from build123d import *

# Parameters (mm, degrees)
SKETCH_2_W          = 130
SKETCH_2_H          = 80
SKETCH_2_R          = 2.5
EXTRUDE_1_DEPTH     = 4.5
SKETCH_4_W          = 80
SKETCH_4_H          = 70
EXTRUDE_2_DEPTH     = 4.5
SKETCH_6_R          = 1.15
CUT_EXTRUDE_2_DEPTH = 4.5
SKETCH_7_R          = 1.15
CUT_EXTRUDE_3_DEPTH = 4.5
SKETCH_8_R          = 1.35
CUT_EXTRUDE_4_DEPTH = 10
SKETCH_9_W          = 40
SKETCH_9_H          = 10
SKETCH_9_W_2        = 30
CUT_EXTRUDE_5_DEPTH = 10
SKETCH_11_W         = 50
SKETCH_11_H         = 30
EXTRUDE_3_DEPTH     = 4.5
SKETCH_12_W         = 20
SKETCH_12_H         = 15
CUT_EXTRUDE_6_DEPTH = 10
SKETCH_13_R         = 2
CUT_EXTRUDE_7_DEPTH = 10
SKETCH_14_R         = 2
CUT_EXTRUDE_8_DEPTH = 10
SKETCH_15_W         = 15
SKETCH_15_H         = 40
CUT_EXTRUDE_9_DEPTH = 10


with BuildPart() as part:
    # 草图2 → 凸台-拉伸1 (new body)
    with BuildSketch(Plane(origin=(0, 0, 0), x_dir=(1, 0, 0), z_dir=(0, 1, 0))):
        with Locations((0, 15)):
            Rectangle(SKETCH_2_W, SKETCH_2_H)
        with Locations(Location((-57, 47, 0), (0, 0, 270))):
            Circle(SKETCH_2_R, mode=Mode.SUBTRACT)
        with Locations(Location((57, 47, 0), (0, 0, 90))):
            Circle(SKETCH_2_R, mode=Mode.SUBTRACT)
        with Locations(Location((57, -17, 0), (0, 0, 270))):
            Circle(SKETCH_2_R, mode=Mode.SUBTRACT)
        with Locations(Location((-57, -17, 0), (0, 0, 90))):
            Circle(SKETCH_2_R, mode=Mode.SUBTRACT)
    extrude(amount=EXTRUDE_1_DEPTH)

    # 草图4 → 凸台-拉伸2 (add)
    with BuildSketch(Plane.XZ):
        with Locations((0, 60)):
            Rectangle(SKETCH_4_W, SKETCH_4_H)
    extrude(amount=-EXTRUDE_2_DEPTH)

    # 草图6 → 切除-拉伸2 (cut)
    with BuildSketch(Plane.XZ):
        with Locations(Location((-31, 5.56384156, 0), (0, 0, 270))):
            Circle(SKETCH_6_R)
        with Locations(Location((31, 5.56384156, 0), (0, 0, 270))):
            Circle(SKETCH_6_R)
    extrude(amount=-CUT_EXTRUDE_2_DEPTH, mode=Mode.SUBTRACT)

    # 草图7 → 切除-拉伸3 (cut)
    with BuildSketch(Plane.XZ):
        with Locations(Location((31, 5.56384156, 0), (0, 0, 270))):
            Circle(SKETCH_7_R)
        with Locations(Location((-25, -51.43615844, 0), (0, 0, 270))):
            Circle(SKETCH_7_R)
        with Locations(Location((25, -51.43615844, 0), (0, 0, 270))):
            Circle(SKETCH_7_R)
    extrude(amount=-CUT_EXTRUDE_3_DEPTH, mode=Mode.SUBTRACT)

    # 草图8 → 切除-拉伸4 (cut)
    with BuildSketch(Plane.XZ):
        with Locations(Location((-21.50477, 84.936614939, 0), (0, 0, 270))):
            Circle(SKETCH_8_R)
        with Locations(Location((36.4733, 84.920764939, 0), (0, 0, 270))):
            Circle(SKETCH_8_R)
        with Locations(Location((36.4823, 35.933764939, 0), (0, 0, 270))):
            Circle(SKETCH_8_R)
        with Locations(Location((-21.5077, 35.922764939, 0), (0, 0, 270))):
            Circle(SKETCH_8_R)
    extrude(amount=-CUT_EXTRUDE_4_DEPTH, mode=Mode.SUBTRACT)

    # 草图9 → 切除-拉伸5 (cut)
    with BuildSketch(Plane.XZ):
        with Locations((0, -5.362073184)):
            Rectangle(SKETCH_9_W, SKETCH_9_H)
        with Locations((0, -28.22464148)):
            Rectangle(SKETCH_9_W, SKETCH_9_H)
        with Locations((7, 71.526054591)):
            Rectangle(SKETCH_9_W_2, SKETCH_9_H)
        with Locations((7, 52.012779739)):
            Rectangle(SKETCH_9_W_2, SKETCH_9_H)
    extrude(amount=-CUT_EXTRUDE_5_DEPTH, mode=Mode.SUBTRACT)

    # 草图11 → 凸台-拉伸3 (add)
    with BuildSketch(Plane.XZ):
        with Locations((0, -70)):
            Rectangle(SKETCH_11_W, SKETCH_11_H)
    extrude(amount=-EXTRUDE_3_DEPTH)

    # 草图12 → 切除-拉伸6 (cut)
    with BuildSketch(Plane.XZ):
        with Locations((0, -67.5)):
            Rectangle(SKETCH_12_W, SKETCH_12_H)
    extrude(amount=-CUT_EXTRUDE_6_DEPTH, mode=Mode.SUBTRACT)

    # 草图13 → 切除-拉伸7 (cut)
    with BuildSketch(Plane.XZ):
        with Locations(Location((-57, 8, 0), (0, 0, 270))):
            Circle(SKETCH_13_R)
        with Locations(Location((-57, -38, 0), (0, 0, 270))):
            Circle(SKETCH_13_R)
        with Locations(Location((-33, -38, 0), (0, 0, 270))):
            Circle(SKETCH_13_R)
    extrude(amount=-CUT_EXTRUDE_7_DEPTH, mode=Mode.SUBTRACT)

    # 草图14 → 切除-拉伸8 (cut)
    with BuildSketch(Plane.XZ):
        with Locations(Location((-35, -27, 0), (0, 0, 270))):
            Circle(SKETCH_14_R)
        with Locations(Location((-35, -3, 0), (0, 0, 270))):
            Circle(SKETCH_14_R)
    extrude(amount=-CUT_EXTRUDE_8_DEPTH, mode=Mode.SUBTRACT)

    # 草图15 → 切除-拉伸9 (cut)
    with BuildSketch(Plane.XZ):
        with Locations((47.5, -15)):
            Rectangle(SKETCH_15_W, SKETCH_15_H)
    extrude(amount=-CUT_EXTRUDE_9_DEPTH, mode=Mode.SUBTRACT)


solid = part.part
Verification items for the finished model (mm, model axes). A direction names the side the tool comes from. Give positions to 0.01 mm unless a question says otherwise; leave off trailing zeros. Write each loop counter-clockwise with the first axis right and the second up, starting at its lowest first coordinate (ties: lowest second). Pieces come first, ordered by that corner, then holes.
(1) Material ranges on line 1 (Z direction, x = 16, y = 2.6); line 2 (X direction, y = 3.25, z = -3); line 3 (Z direction, x = -56, y = 1.8), recorded low to high.
(2) Access from +Z, -Z, +X, -X, +Y, -Y to the whole of each face (thin tool, end or side, straight path). Record for faces 4 (the face through (55, 2, -15)), 5 (the face through (-53, 2, 25)), 6 (the face through (-1, 2, 95)).
(3) Gauge pin test, flat ends, axial feed: pin 1 (2 mm diameter, centred on y = 2, z = -69.5, fed in from +X); pin 2 (2 mm diameter, centred on x = 57.5, y = 2, fed in from +Z). Record the tip position at first contact, or that the pin passes through.
(4) Cross-section at C-C (x = 57). Enter the section's corners in (y, z), plus the area to 3 significant figures.
(5) Cross-section at A-A (z = -27). Enter the section's corners in (x, y).
(6) Cross-section at B-B (z = -47). Enter the section's corners in (x, y), plus the area to 3 significant figures.
(7) Cross-section at D-D (x = -57). Enter the section's corners in (y, z), plus the area to 3 significant figures.
(8) Mould release check, pull along X, two halves, no side actions. Record for faces 1 (the face through (22, 2, 71)), 2 (the face through (-8, 2, 71)), 3 (the face through (-1, 0, 4)): +X half, -X half, draft (parallel to the pull), parting line (faces both ways), or undercut.
Worked out:
1. line 1: z = -85 to -33.22, -23.22 to -10.36, -0.36 to 47.01, 57.01 to 66.53, 76.53 to 95
1. line 2: x = -65 to -37, -33 to -20, 20 to 40, 55 to 65
1. line 3: z = -55 to -49.29, -44.71 to -39.73, -36.27 to 6.27, 9.73 to 14.71, 19.29 to 25
2. face 4: +Y, -Y
2. face 5: +Z, -X, +Y, -Y
2. face 6: +Z, +X, -X, +Y, -Y
3. pin 1: stops at x = 25
3. pin 2: stops at z = 25
4. outline: (0, -55) - (4.5, -55) - (4.5, -49.5) - (0, -49.5) - close; (0, -44.5) - (4.5, -44.5) - (4.5, 14.5) - (0, 14.5) - close; (0, 19.5) - (4.5, 19.5) - (4.5, 25) - (0, 25) - close
4. area: 315 mm2
5. outline: (-65, 0) - (-37, 0) - (-37, 4.5) - (-65, 4.5) - close; (-33, 0) - (-20, 0) - (-20, 4.5) - (-33, 4.5) - close; (20, 0) - (40, 0) - (40, 4.5) - (20, 4.5) - close; (55, 0) - (65, 0) - (65, 4.5) - (55, 4.5) - close
6. outline: (-65, 0) - (-59.5, 0) - (-59.5, 4.5) - (-65, 4.5) - close; (-54.5, 0) - (54.5, 0) - (54.5, 4.5) - (-54.5, 4.5) - close; (59.5, 0) - (65, 0) - (65, 4.5) - (59.5, 4.5) - close
6. area: 540 mm2
7. outline: (0, -55) - (4.5, -55) - (4.5, -49.5) - (0, -49.5) - close; (0, -44.5) - (4.5, -44.5) - (4.5, -40) - (0, -40) - close; (0, -36) - (4.5, -36) - (4.5, 6) - (0, 6) - close; (0, 10) - (4.5, 10) - (4.5, 14.5) - (0, 14.5) - close; (0, 19.5) - (4.5, 19.5) - (4.5, 25) - (0, 25) - close
7. area: 279 mm2
8. face 1: undercut
8. face 2: undercut
8. face 3: draft
